Part print with two shaded views. Sizes in mm from the minimum x, y, z corner. Give positions to 0.01 mm unless a question says otherwise; leave off trailing zeros. Write each loop counter-clockwise with the first axis right and the second up, starting at its lowest first coordinate (ties: lowest second). Pieces come first, ordered by that corner, then holes. Notation, with made-up numbers: (-23.5, 9) -> (-8.5, 9) arc R11 cw to (-8.5, 15) -> close; hole circle Ø2 at (-18.5, -11.75). An arc over 180 degrees is marked (long way). Use one line per item in the form item = value. Start each with the question number.
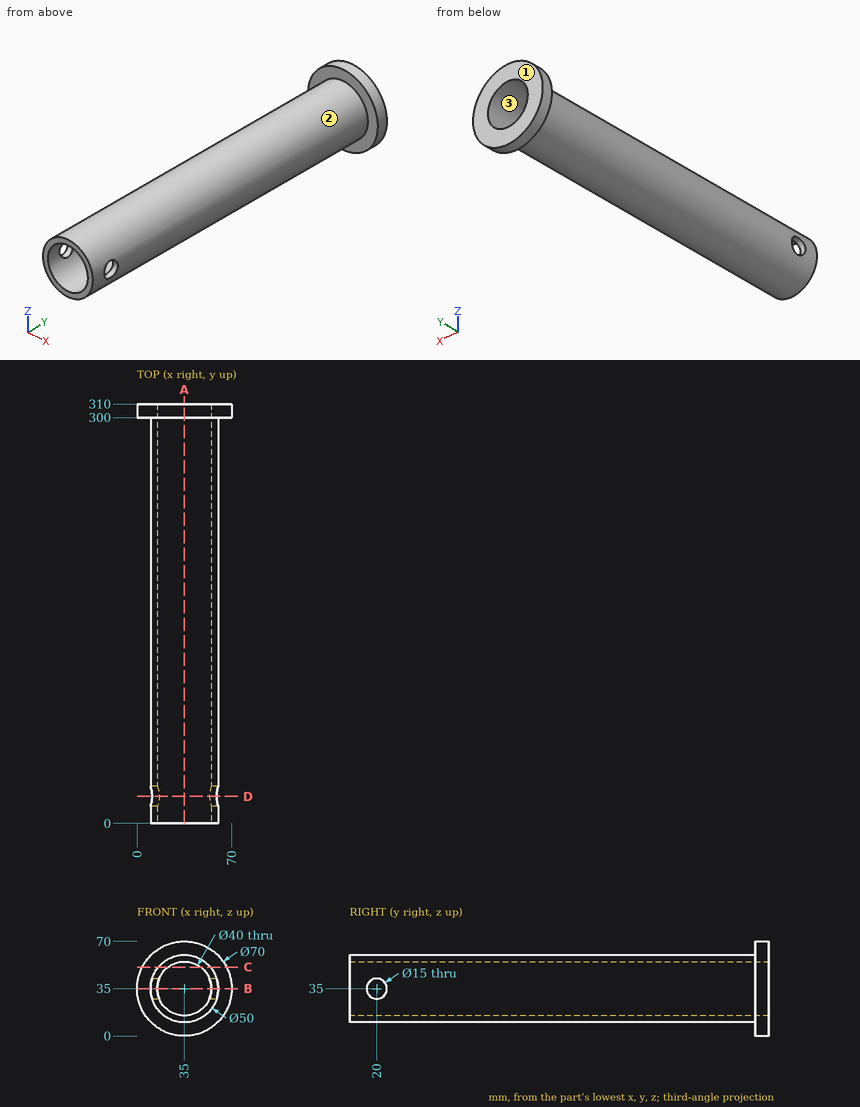
1) Cut at B-B (z = 35). Give the cut face in (x, y).
2) Cut at D-D (y = 20). Give the cut face in (x, z), and give its area (3 significant figures).
3) Two-plate mould, pull along X, no slides. Class the marked faces 1, 2 and 3: released by +X, released by -X, zero draft, split by the parting line, or undercut.
4) Cut at C-C (z = 51). Give the cut face in (x, y), and give its area (3 significant figures).
5) Wall check: line 1 along X through (y, z) = (246.5, 35); line 2 along Y through (x, z) = (58, 35); line 3 along Y through (x, z) = (20, 66). Give the ranges that are in metal, low to high. Write a range as from..to.
6) Cut at A-A (x = 35). Give the cut face in (y, z), and give its area (3 significant figures).
7) Pin check, flat tips, straight feed: pin 1 (2 mm diameter, centred on x = 15, y = 167, fed in from +Z); pin 2 (8 mm diameter, centred on x = 45, y = 70, fed in from -Z); pin 3 (4 mm diameter, centred on x = 12.5, y = 187.5, fed in from -Z). Stop position of each tip, or through.
Final values:
q1.outline = (0, 300) -> (10, 300) -> (10, 27.5) -> (15, 27.5) -> (15, 310) -> (0, 310) -> close; (10, 0) -> (15, 0) -> (15, 12.5) -> (10, 12.5) -> close; (55, 0) -> (60, 0) -> (60, 12.5) -> (55, 12.5) -> close; (55, 27.5) -> (60, 27.5) -> (60, 300) -> (70, 300) -> (70, 310) -> (55, 310) -> close
q2.outline = (11.15, 27.5) arc R25 ccw to (58.85, 27.5) -> (53.54, 27.5) arc R20 cw to (16.46, 27.5) -> close; (11.15, 42.5) -> (16.46, 42.5) arc R20 cw to (53.54, 42.5) -> (58.85, 42.5) arc R25 ccw to start
q2.area = 554 mm^2
q3.face_1 = zero draft
q3.face_2 = split by the parting line
q3.face_3 = undercut
q4.outline = (3.87, 300) -> (15.79, 300) -> (15.79, 0) -> (23, 0) -> (23, 310) -> (3.87, 310) -> close; (47, 0) -> (54.21, 0) -> (54.21, 300) -> (66.13, 300) -> (66.13, 310) -> (47, 310) -> close
q4.area = 4,710 mm^2
q5.line_1 = 10..15, 55..60
q5.line_2 = 0..12.5, 27.5..310
q5.line_3 = 300..310
q6.outline = (0, 10) -> (300, 10) -> (300, 0) -> (310, 0) -> (310, 15) -> (0, 15) -> close; (0, 55) -> (310, 55) -> (310, 70) -> (300, 70) -> (300, 60) -> (0, 60) -> close
q6.area = 3,300 mm^2
q7.pin_1 = 51.25
q7.pin_2 = 10.73
q7.pin_3 = 20.69
